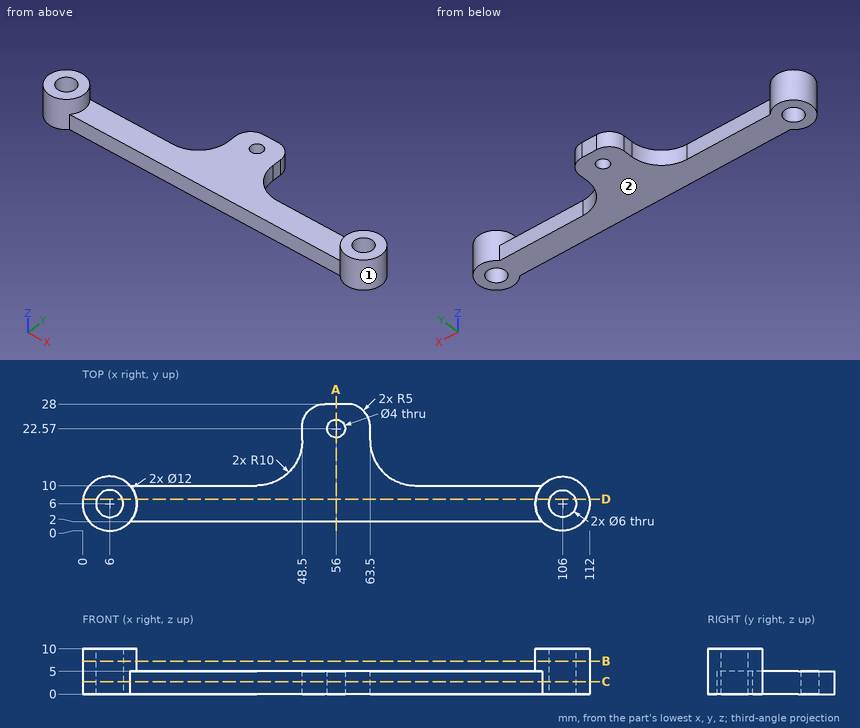
The figure shows three views and two pictorial views of one solid part (mm, origin at its lowest corner). Answer the questions. Round coordinates to 2 decimals unless told otherwise and drop trailing zeros. Order: outer loops, then holes, each group sorted by start corner. A loop starts at its lowest first (then second) coordinate and runs counter-clockwise, first axis right, second up. Notation, with made-up numbers: (-20.5, 13) - (33.5, 13) arc R21 cw to (33.5, 22) - close; hole circle Ø1 at (1.25, -23). An arc over 180 degrees is marked (long way). Write item = value, one per line. Start each with the question number.
1) Section C-C, the plane z = 2.75 is taken. Write down the section's boundary in (x, y).
2) Straight lines are drawn through the part: L1, parallel to Y at x = 6, z = 4.5; L2, parallel to Y at x = 56, z = 2.3; L3, parallel to Z at x = 53, y = 10.75. For each, find the intervals that lie inside material, in ascending order.
3) Given pin 1 (5.5 mm diameter, centred on x = 77.5, z = 2, fed in from -Y); pin 2 (10 mm diameter, centred on x = 64.5, y = 20, fed in from -Z); pin 3 (1.5 mm diameter, centred on x = 81, z = 2.5, fed in from +Y); pin 4 (1.5 mm diameter, centred on y = 21.5, z = 2, fed in from -X), each flat-ended and moving along its own axis, determine where each tip first touches the part or whether it passes through.
4) Section A-A, the plane x = 56 is taken. Write down the section's boundary in (y, z), plus the area to 3 significant figures.
5) Section B-B, the plane z = 7.25 is taken. Write down the section's boundary in (x, y), plus the area to 3 significant figures.
6) Section D-D, the plane y = 7 is taken. Write down the section's boundary in (x, z), plus the area to 3 significant figures.
7) For a pull along X with two mould halves and no side action, classify the marked faces 1 and 2 as released by +X, released by -X, zero draft, split by the parting line, or undercut.
Results list:
q1.outline = (10.47, 2) - (101.53, 2) arc R6 ccw (long way) to (101.53, 10) - (73.5, 10) arc R10 cw to (63.5, 20) - (63.5, 23) arc R5 ccw to (58.5, 28) - (53.5, 28) arc R5 ccw to (48.5, 23) - (48.5, 20) arc R10 cw to (38.5, 10) - (10.47, 10) arc R6 ccw (long way) to start; hole circle Ø6 at (6, 6); hole circle Ø4 at (56, 22.57); hole circle Ø6 at (106, 6)
q2.L1 = 0 to 3, 9 to 12
q2.L2 = 2 to 20.57, 24.57 to 28
q2.L3 = 0 to 5
q3.pin_1 = 2
q3.pin_2 = 0
q3.pin_3 = 10
q3.pin_4 = 48.5
q4.outline = (2, 0) - (20.57, 0) - (20.57, 5) - (2, 5) - close; (24.57, 0) - (28, 0) - (28, 5) - (24.57, 5) - close
q4.area = 110 mm^2
q5.outline = circle Ø12 at (6, 6); circle Ø12 at (106, 6); hole circle Ø6 at (6, 6); hole circle Ø6 at (106, 6)
q5.area = 170 mm^2
q6.outline = (0.08, 0) - (3.17, 0) - (3.17, 10) - (0.08, 10) - close; (8.83, 0) - (103.17, 0) - (103.17, 10) - (100.08, 10) - (100.08, 5) - (11.92, 5) - (11.92, 10) - (8.83, 10) - close; (108.83, 0) - (111.92, 0) - (111.92, 10) - (108.83, 10) - close
q6.area = 564 mm^2
q7.face_1 = undercut
q7.face_2 = zero draft
